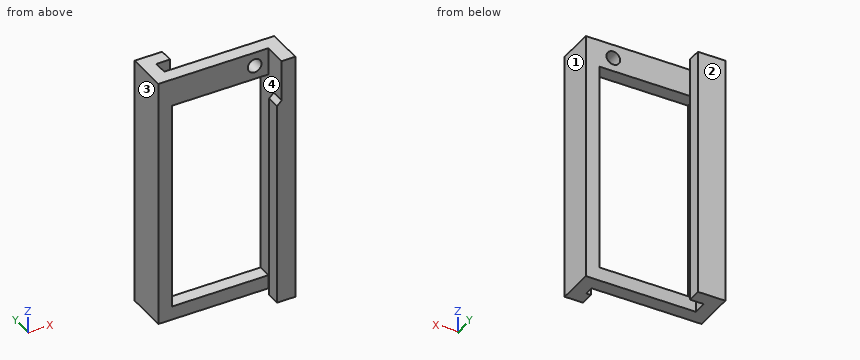
from build123d import *

# Parameters (mm, degrees)
F1_DEPTH = 55
F2_R     = 1.5
F2_W     = 21
F2_H     = 46
F3_DEPTH = 5
F4_W     = 3
F4_H     = 10
F5_DEPTH = 1
F6_SIZE  = 0.99999


# Not quite as in the source:
# - a fillet or chamfer is up to 0.001 mm smaller than in the source, because OpenCascade refuses the exact size


with BuildPart() as f1:
    # F0 (on Top) → F1 (new body)
    with BuildSketch(Plane.XY):
        Polygon((24, 0), (0, 0), (0, 2.9999995536), (3, 2.9999995536), (3, 5.9999995536), (-3, 5.9999995536), (-3, -3.0000002232), (21, -3.0000002232), (21, -5.0000002232), (20, -5.0000002232), (20, -8.0000002232), (24, -8.0000002232), align=None)
    extrude(amount=F1_DEPTH)

    # F2 (on face) → F3 (cut)
    with BuildSketch(Plane.XZ.offset(3.0000002232)):
        with Locations((18, 52)):
            Circle(F2_R)
        with Locations((10.5, 26)):
            Rectangle(F2_W, F2_H)
    extrude(amount=-F3_DEPTH, mode=Mode.SUBTRACT)

    # F4 (on face) → F5 (cut)
    with BuildSketch(Plane(origin=(20, 0, 0), x_dir=(0, -1, 0), z_dir=(-1, 0, 0))):
        with Locations((6.5000002232, 50)):
            Rectangle(F4_W, F4_H)
    extrude(amount=-F5_DEPTH, mode=Mode.SUBTRACT)

    # F6 (size 1 in the source; OpenCascade refuses exactly that, so slightly less here)
    f6_edges = [f1.edges().sort_by_distance(p)[0] for p in [
        (21, -6.5, 45),
    ]]
    chamfer(f6_edges, length=F6_SIZE)


solid = f1.part
Geometry check sheet. Reference: the model listing, model coordinates, mm. Face numbers are marked on the shaded views. Coordinates: 2 decimals unless noted, no trailing zeros. Order: outer loops, then holes, each group sorted by start corner. A loop starts at its lowest first (then second) coordinate and runs counter-clockwise, first axis right, second up. Notation, with made-up numbers: (83.5, 17.5) - (133.5, 17.5) arc R21 ccw to (133.5, 50.5) - close; hole circle Ø6 at (-12.5, 20). An arc over 180 degrees is marked (long way). One line per item, written item: value.
(1) Thickness scan on probe 1 along Z at (x, y) = (18, -1.05); probe 2 along X at (y, z) = (-0.75, 46); probe 3 along X at (y, z) = (-3.75, 20.5). Record the ranges inside material, lowest first. Write a range as from..to.
Data:
probe 1: z = 0..3, 49..50.5, 53.5..55
probe 2: x = -3..0, 21..24
probe 3: x = 21..24
(2) Release check for a two-part mould opening along X. For the marked faces 1, 2, 3 and 4 record: +X half, -X half, draft (parallel to the pull), parting line (faces both ways), or undercut.
Data:
face 1: +X half
face 2: draft
face 3: -X half
face 4: undercut
(3) Depth check by flat-ended pin: pin 1 Ø3.5 at (y, z) = (4.5, 20) entering from +X; pin 2 Ø5 at (x, y) = (4, 0) entering from -Z; pin 3 Ø3.5 at (x, z) = (18, 52) entering from +Y; pin 4 Ø12 at (x, z) = (3.5, 20) entering from -Y. Enter the tip coordinate at first touch or a pass-through.
Data:
pin 1: stops at x = 3
pin 2: stops at z = 0
pin 3: stops at y = 0
pin 4: stops at y = -3
(4) Sectioned sample at A-A (x = 18). Enter the section's corners in (y, z), and give its area (3 significant figures).
Data:
outline: (-3, 0) - (0, 0) - (0, 3) - (-3, 3) - close; (-3, 49) - (0, 49) - (0, 50.5) - (-3, 50.5) - close; (-3, 53.5) - (0, 53.5) - (0, 55) - (-3, 55) - close
area: 18.0 mm^2
(5) Sectioned sample at D-D (x = 4.25). Enter the section's corners in (y, z).
Data:
outline: (-3, 0) - (0, 0) - (0, 3) - (-3, 3) - close; (-3, 49) - (0, 49) - (0, 55) - (-3, 55) - close
(6) Sectioned sample at C-C (y = -1). Enter the section's corners in (x, z).
Data:
outline: (-3, 0) - (24, 0) - (24, 55) - (-3, 55) - close; hole (0, 3) - (21, 3) - (21, 49) - (0, 49) - close; hole circle Ø3 at (18, 52)
(7) Sectioned sample at B-B (z = 23). Enter the section's corners in (x, y), and give its area (3 significant figures).
Data:
outline: (-3, -3) - (0, -3) - (0, 3) - (3, 3) - (3, 6) - (-3, 6) - close; (20, -8) - (24, -8) - (24, 0) - (21, 0) - (21, -5) - (20, -5) - close
area: 63.0 mm^2
